Answer from the drawing. Dimensions are ordinates in mm from the lowest x, y and z of the part. A direction names the side the tool comes from. Coordinates: 2 decimals unless noted, no trailing zeros. Loops run counter-clockwise (first coordinate to the right, second up) from the corner with the lowest first, then second, coordinate; pieces in that order, holes last. Notation, with made-up numbers: M -32.5,-25.5 L 12.5,-25.5 A20 cw 12.5,-2.5 Z; hole C -6,26 d5. An arc over 180 degrees is marked long. Put each result on its own line as item: value.
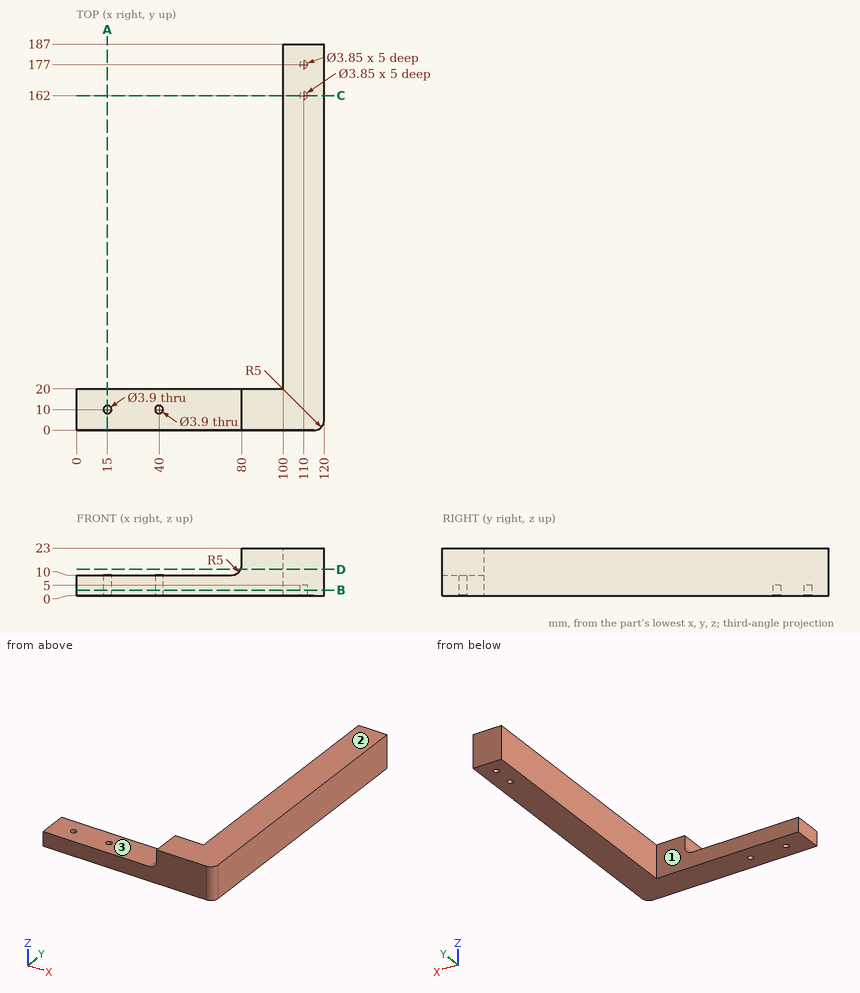
1) Find section D-D, the plane z = 12.75. Write down the section's boundary in (x, y).
Answer list:
outline: M 79.47,0 L 115,0 A5 ccw 120,5 L 120,187 L 100,187 L 100,20 L 79.47,20 Z
2) Straight lines are drawn through the part: line 1 (Y direction, x = 110, z = 2.3) (3 decimals); line 2 (Y direction, x = 15, z = 2.5); line 3 (X direction, y = 162, z = 2.8) (3 decimals). For each, find the intervals that lie inside material, in ascending order. Write a range as [from, to].
Answer list:
line 1: y = [0, 160.075], [163.925, 175.075], [178.925, 187]
line 2: y = [0, 8.05], [11.95, 20]
line 3: x = [100, 108.075], [111.925, 120]
3) Given pin 1 Ø1 at (y, z) = (51, 8) entering from -X; pin 2 Ø6 at (x, y) = (110, 162) entering from -Z; pin 3 Ø6.5 at (y, z) = (6.5, 20) entering from -X; pin 4 Ø22 at (x, y) = (54, 7) entering from +Z, each flat-ended and moving along its own axis, determine where each tip first touches the part or whether it passes through.
Answer list:
pin 1: stops at x = 100
pin 2: stops at z = 0
pin 3: stops at x = 80
pin 4: stops at z = 10
4) Find section C-C, the plane y = 162. Write down the section's boundary in (x, z) (3 decimals).
Answer list:
outline: M 100,0 L 108.075,0 L 108.075,5 L 111.925,5 L 111.925,0 L 120,0 L 120,23 L 100,23 Z
5) Which of the six approach directions +Z, -Z, +X, -X, +Y, -Y give full straight-line access (tool end or side, diameter ignored) to the marked faces 1, 2 and 3?
Answer list:
face 1: +Z, -Z, -X, +Y
face 2: +Z, +X, -X, +Y, -Y
face 3: +Z, -X, +Y, -Y
6) Find section A-A, the plane x = 15. Write down the section's boundary in (y, z).
Answer list:
outline: M 0,0 L 8.05,0 L 8.05,10 L 0,10 Z; M 11.95,0 L 20,0 L 20,10 L 11.95,10 Z
7) Find section B-B, the plane z = 2.75. Write down the section's boundary in (x, y) (3 decimals), plus the area to 3 significant figures.
Answer list:
outline: M 0,0 L 115,0 A5 ccw 120,5 L 120,187 L 100,187 L 100,20 L 0,20 Z; hole C 15,10 d3.9; hole C 40,10 d3.9; hole C 110,162 d3.85; hole C 110,177 d3.85
area: 5,690 mm^2
